Verification items for the finished model (mm, model axes). A direction names the side the tool comes from. Give positions to 0.01 mm unless a question says otherwise; leave off trailing zeros. Order: outer loops, then holes, each group sorted by start corner. A loop starts at its lowest first (then second) coordinate and runs counter-clockwise, first axis right, second up.
(1) Sectioned sample at B-B on x = -26.5. Record the cut outline in (y, z), plus the area to 3 significant figures.
(2) Gauge pin test, flat ends, axial feed: pin 1 (3 mm diameter, centred on y = 7, z = 4.5, fed in from -X); pin 2 (1.7 mm diameter, centred on x = -1, z = 5, fed in from +Y); pin 3 (1.7 mm diameter, centred on x = -31.5, z = 7, fed in from -Y). Record the tip position at first contact, or that the pin passes through.
(3) Sectioned sample at C-C on y = 25. Record the cut outline in (x, z), plus the area to 3 significant figures.
(4) Sectioned sample at D-D on x = 14. Record the cut outline in (y, z).
(5) Sectioned sample at A-A on z = 4.5. Count the separate pieces of the cut face and the enclosed holes in it, plus the area to 3 significant figures.
(6) Mould release check, pull along X, two halves, no side actions. Record for faces 4 (the face through (-8.745, 34, 5)), 5 (the face through (-20.852, -9.654, 5.07)), 6 (the face through (-23, -1.847, 5)), 7 (the face through (-16, -3, 10)): pulls with the +X half, pulls with the -X half, needs draft (parallel to the pull), parting line crosses it, or undercut.
(7) Scan lines: L1, parallel to Y at x = -36.3, z = 4.5; L2, parallel to Y at x = -30.5, z = 4.5; L3, parallel to X at y = -8.5, z = 9. Record each from-to range of solid material in increasing order.
(8) Access from +Z, -Z, +X, -X, +Y, -Y to the whole of each face (thin tool, end or side, straight path). Record for faces 1 (the face through (5, -10.19, 5)), 2 (the face through (-18, -17, 5)), 3 (the face through (0, -4.796, 5)).
```python
from build123d import *

# Parameters (mm, degrees)
BOSS_EXTRUDE1_DEPTH = 10
CUT_EXTRUDE1_REACH  = 70.061
SKETCH2_R           = 3
FILLET1_R           = 10
FILLET2_R           = 5


with BuildPart() as part:
    # Sketch1 → Boss-Extrude1 (new body)
    with BuildSketch(Plane.XY):
        with BuildLine():
            Line((-10.5918, -13), (-4.305880552, -13))
            Line((-4.305880552, -13), (-4.287512407, -13))
            ThreePointArc((-4.287512407, -13), (-3.333616586, -12.604883414), (-2.9385, -11.650987593))
            Line((-2.9385, -11.650987593), (-2.9385, -11.539212407))
            ThreePointArc((-2.9385, -11.539212407), (-3.333616586, -10.585316586), (-4.287512407, -10.1902))
            Line((-4.287512407, -10.1902), (-6.416408329, -10.1902))
            ThreePointArc((-6.416408329, -10.1902), (-7.137514675, -9.708134418), (-6.967711912, -8.857517813))
            Line((-6.967711912, -8.857517813), (-3.740331666, -5.636015806))
            ThreePointArc((-3.740331666, -5.636015806), (-2.808257752, -5.01414519), (-1.709253557, -4.7958))
            Line((-1.709253557, -4.7958), (1.709253557, -4.7958))
            ThreePointArc((1.709253557, -4.7958), (2.808257752, -5.01414519), (3.740331666, -5.636015806))
            Line((3.740331666, -5.636015806), (6.967711912, -8.857517813))
            ThreePointArc((6.967711912, -8.857517813), (7.137514675, -9.708134418), (6.416408329, -10.1902))
            Line((6.416408329, -10.1902), (4.287512407, -10.1902))
            ThreePointArc((4.287512407, -10.1902), (3.333616586, -10.585316586), (2.9385, -11.539212407))
            Line((2.9385, -11.539212407), (2.9385, -11.650987593))
            ThreePointArc((2.9385, -11.650987593), (3.333616586, -12.604883414), (4.287512407, -13))
            Line((4.287512407, -13), (5.321597603, -13))
            Line((5.321597603, -13), (10.5918, -13))
            ThreePointArc((10.5918, -13), (12.29465455, -12.29465455), (13, -10.5918))
            Line((13, -10.5918), (13, -5.3170836))
            Line((13, -5.3170836), (13, -4.287469289))
            ThreePointArc((13, -4.287469289), (12.604883414, -3.333573468), (11.650987593, -2.938456882))
            Line((11.650987593, -2.938456882), (11.539212407, -2.938456882))
            ThreePointArc((11.539212407, -2.938456882), (10.585316586, -3.333573468), (10.1902, -4.287469289))
            Line((10.1902, -4.287469289), (10.1902, -6.402089023))
            ThreePointArc((10.1902, -6.402089023), (9.74154152, -7.073969797), (8.94902056, -6.917034355))
            Line((8.94902056, -6.917034355), (5.652895046, -3.628441884))
            ThreePointArc((5.652895046, -3.628441884), (5.027976112, -2.694919539), (4.8085, -1.593185507))
            Line((4.8085, -1.593185507), (4.8085, 1.593185507))
            ThreePointArc((4.8085, 1.593185507), (5.027976112, 2.694919539), (5.652895046, 3.628441884))
            Line((5.652895046, 3.628441884), (8.94902056, 6.917034355))
            ThreePointArc((8.94902056, 6.917034355), (9.74154152, 7.073969797), (10.1902, 6.402089023))
            Line((10.1902, 6.402089023), (10.1902, 4.287469289))
            ThreePointArc((10.1902, 4.287469289), (10.585316586, 3.333573468), (11.539212407, 2.938456882))
            Line((11.539212407, 2.938456882), (11.650987593, 2.938456882))
            ThreePointArc((11.650987593, 2.938456882), (12.604883414, 3.333573468), (13, 4.287469289))
            Line((13, 4.287469289), (13, 5.3170836))
            Line((13, 5.3170836), (13, 7.9544418))
            Line((13, 7.9544418), (18, 7.9544418))
            Line((18, 7.9544418), (18, -18))
            Line((18, -18), (-18, -18))
            Line((-18, -18), (-18, -6.6473334))
            Line((-18, -6.6473334), (-38.6, -6.6473334))
            Line((-38.6, -6.6473334), (-38.6, 36.4526666))
            Line((-38.6, 36.4526666), (-8.745302284, 36.4526666))
            Line((-8.745302284, 36.4526666), (-8.745302284, 31.4526666))
            Line((-8.745302284, 31.4526666), (-33.6, 31.4526666))
            Line((-33.6, 31.4526666), (-33.6, -1.8473334))
            Line((-33.6, -1.8473334), (-13, -1.8473334))
            Line((-13, -1.8473334), (-13, -4.287469289))
            Line((-13, -4.287469289), (-13, -10.5918))
            ThreePointArc((-13, -10.5918), (-12.29465455, -12.29465455), (-10.5918, -13))
        make_face()
    extrude(amount=BOSS_EXTRUDE1_DEPTH)

    # Sketch2 → Cut-Extrude1 (cut, up to next)
    with BuildSketch(Plane.ZY.offset(38.6), mode=Mode.PRIVATE) as cut_extrude1_sk1:
        with Locations((4.5, 26.4526666)):
            Circle(SKETCH2_R)
    cut_extrude1_tool1 = extrude(cut_extrude1_sk1.sketch, amount=-CUT_EXTRUDE1_REACH, mode=Mode.PRIVATE) & part.part
    # Sketch2 → Cut-Extrude1 (cut, up to next)
    with BuildSketch(Plane.ZY.offset(38.6), mode=Mode.PRIVATE) as cut_extrude1_sk2:
        with Locations((4.5, 7.9526666)):
            Circle(SKETCH2_R)
    cut_extrude1_tool2 = extrude(cut_extrude1_sk2.sketch, amount=-CUT_EXTRUDE1_REACH, mode=Mode.PRIVATE) & part.part
    add(cut_extrude1_tool1.solids().sort_by_distance((-38.6, 26.452667, 4.5))[0], mode=Mode.SUBTRACT)
    add(cut_extrude1_tool2.solids().sort_by_distance((-38.6, 7.952667, 4.5))[0], mode=Mode.SUBTRACT)

    # Fillet1
    fillet1_edges = [part.edges().sort_by_distance(p)[0] for p in [
        (-18, -6.6473334, 5),
    ]]
    fillet(fillet1_edges, radius=FILLET1_R)

    # Fillet2
    fillet2_edges = [part.edges().sort_by_distance(p)[0] for p in [
        (18, -18, 5),
        (-38.6, -6.6473334, 5),
        (-38.6, 36.4526666, 5),
    ]]
    fillet(fillet2_edges, radius=FILLET2_R)


solid = part.part
```
Ans:
1. outline: (-6.76, 0) - (-1.85, 0) - (-1.85, 10) - (-6.76, 10) - close; (31.45, 0) - (36.45, 0) - (36.45, 10) - (31.45, 10) - close
1. area: 99.1 mm2
2. pin 1: stops at x = 7.53
2. pin 2: stops at y = -4.8
2. pin 3: stops at y = -6.65
3. outline: (-38.6, 0) - (-33.6, 0) - (-33.6, 1.88) - (-38.6, 1.88) - close; (-38.6, 7.12) - (-33.6, 7.12) - (-33.6, 10) - (-38.6, 10) - close
3. area: 23.8 mm2
4. outline: (-17.9, 0) - (7.95, 0) - (7.95, 10) - (-17.9, 10) - close
5. separate pieces: 3
5. enclosed holes: 0
5. area: 855 mm2
6. face 4: pulls with the +X half
6. face 5: pulls with the -X half
6. face 6: undercut
6. face 7: needs draft
7. L1: y = -5.86 to 4.95, 10.95 to 23.45, 29.45 to 35.66
7. L2: y = -6.65 to -1.85, 31.45 to 36.45
7. L3: x = -22.2 to -13, -6.61 to 6.61, 13 to 18
8. face 1: +Z, -Z
8. face 2: +Z, -Z, -X, -Y
8. face 3: +Z, -Z, +Y
